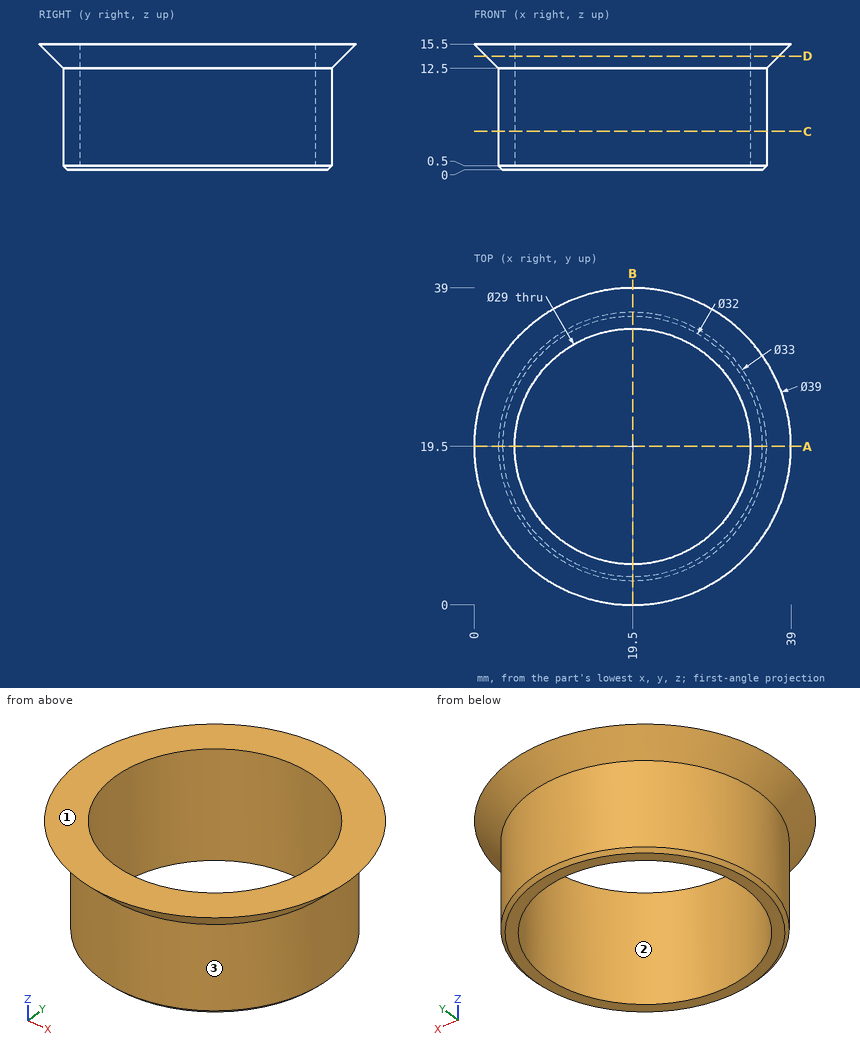
Check sheet for the drawn part. Datum: minimum x, y, z corner. Units: mm. Give positions to 0.01 mm unless a question says otherwise; leave off trailing zeros. Order: outer loops, then holes, each group sorted by start corner. A loop starts at its lowest first (then second) coordinate and runs counter-clockwise, first axis right, second up. Notation, with made-up numbers: (-37.5, -28) - (11.5, -28) arc R11 ccw to (11.5, -7) - close; hole circle Ø7 at (43.25, 55.25). An arc over 180 degrees is marked (long way). Write item = value, one per line. Start each with the question number.
1) Gauge pin test, flat ends, axial feed: pin 1 Ø3 at (y, z) = (14, 3) entering from -X; pin 2 Ø2 at (x, z) = (8.5, 11.5) entering from -Y; pin 3 Ø1.5 at (x, z) = (26, 7) entering from +Y. Record the tip position at first contact, or that the pin passes through.
2) Scan lines: L1, parallel to Y at x = 19.5, z = 11; L2, parallel to X at y = 19, z = 6.5; L3, parallel to Y at x = 28, z = 2.25. Record each from-to range of solid material in increasing order.
3) Section check A-A (y = 19.5). Enter the section's corners in (x, z), then the cut area to 4 significant figures.
4) Draft check along X on the marked faces 1, 2 and 3. Enter one of: released by +X, released by -X, zero draft, split by the parting line, or undercut.
5) Section check C-C (z = 4.75). Enter the section's corners in (x, y).
6) Section check D-D (z = 14). Enter the section's corners in (x, y), then the cut area to 3 significant figures.
Geometry check:
q1.pin_1 = 3.49
q1.pin_2 = 6.38
q1.pin_3 = 34.97
q2.L1 = 3 to 5, 34 to 36
q2.L2 = 3.01 to 5.01, 33.99 to 35.99
q2.L3 = 5.36 to 7.75, 31.25 to 33.64
q3.outline = (0, 15.5) - (3, 12.5) - (3, 0.5) - (3.5, 0) - (5, 0) - (5, 15.5) - close; (34, 0) - (35.5, 0) - (36, 0.5) - (36, 12.5) - (39, 15.5) - (34, 15.5) - close
q3.area = 70.75 mm2
q4.face_1 = zero draft
q4.face_2 = undercut
q4.face_3 = split by the parting line
q5.outline = circle Ø33 at (19.5, 19.5); hole circle Ø29 at (19.5, 19.5)
q6.outline = circle Ø36 at (19.5, 19.5); hole circle Ø29 at (19.5, 19.5)
q6.area = 357 mm2
